Read the model definition and answer for the solid it produces. Units are mm, in the model's axes. A direction names the side the tool comes from. Give positions to 0.01 mm unless a question says otherwise; leave off trailing zeros. Order: outer loops, then holes, each group sorted by start corner. A loop starts at its lowest first (then second) coordinate and runs counter-clockwise, first axis right, second up.
Item 1: A cutting plane is placed at B-B (x = -72.5). Write down the section's boundary in (y, z).
Item 2: The mould has two halves that part along X. Classify faces 4 (the face through (-147.5, 6.18, -0.16)), 5 (the face through (-2, 0, 0)), 6 (the face through (141, 1.5, 0)): +X half, -X half, draft (parallel to the pull), parting line (faces both ways), or undercut.
Item 3: Given pin 1 Ø5 at (y, z) = (8, -3.5) entering from -X; pin 2 Ø1 at (x, y) = (-93.5, 2.5) entering from -Z; pin 3 Ø6 at (x, z) = (135.5, 1.5) entering from +Y, each flat-ended and moving along its own axis, determine where each tip first touches the part or whether it passes through.
Item 4: Which of the six approach directions +Z, -Z, +X, -X, +Y, -Y give full straight-line access (tool end or side, diameter ignored) to faces 1 (the face through (2, 6, -7.5)), 2 (the face through (147.5, 6.18, 0.16)), 3 (the face through (146.445, 6.923, -0.846))?
Item 5: A cutting plane is placed at A-A (y = 6.5). Write down the section's boundary in (x, z).
Item 6: Find the intervals of material crossed by line 1 along X through (y, z) = (9.75, 0); line 2 along Z through (x, y) = (-78.5, 6.5); line 3 along X through (y, z) = (1.25, 0), in increasing order.
from build123d import *

# Parameters (mm, degrees)
BOSS_EXTRUDE1_DEPTH = 1.5
SKETCH2_R           = 6.5
BOSS_EXTRUDE2_DEPTH = 10
BOSS_EXTRUDE3_DEPTH = 1
FILLET1_R           = 2
FILLET2_R           = 1
FILLET3_R           = 1
CUT_EXTRUDE1_DEPTH  = 151.73486657
SKETCH5_R           = 0.75
CUT_EXTRUDE2_DEPTH  = 151.73486657


with BuildPart() as part:
    # Sketch1 → Boss-Extrude1 (new body)
    with BuildSketch(Plane(origin=(0, 0, 0), x_dir=(1, 0, 0), z_dir=(0, 1, 0))):
        with BuildLine():
            Line((140, 7.5), (-140, 7.5))
            ThreePointArc((-140, 7.5), (-147.5, 0), (-140, -7.5))
            Line((-140, -7.5), (140, -7.5))
            ThreePointArc((140, -7.5), (147.5, 0), (140, 7.5))
        make_face()
    extrude(amount=BOSS_EXTRUDE1_DEPTH)

    # Sketch2 → Boss-Extrude2 (add)
    with BuildSketch(Plane(origin=(0, 1.5, 0), x_dir=(1, 0, 0), z_dir=(0, 1, 0))):
        with BuildLine():
            Line((-140, -7.5), (140, -7.5))
            ThreePointArc((140, -7.5), (147.5, 0), (140, 7.5))
            Line((140, 7.5), (-140, 7.5))
            ThreePointArc((-140, 7.5), (-147.5, 0), (-140, -7.5))
        make_face()
        with Locations(Location((140, 0, 0), (0, 0, 270))):
            Circle(SKETCH2_R, mode=Mode.SUBTRACT)
        with BuildLine():
            Line((-140, 6.5), (136.258342613, 6.5))
            ThreePointArc((136.258342613, 6.5), (132.5, 0), (136.258342613, -6.5))
            Line((136.258342613, -6.5), (-140, -6.5))
            ThreePointArc((-140, -6.5), (-146.5, 0), (-140, 6.5))
        make_face(mode=Mode.SUBTRACT)
    extrude(amount=BOSS_EXTRUDE2_DEPTH)

    # Sketch3 → Boss-Extrude3 (add)
    with BuildSketch(Plane(origin=(0, 11.5, 0), x_dir=(1, 0, 0), z_dir=(0, 1, 0))):
        with BuildLine():
            Line((-140, 10), (140, 10))
            ThreePointArc((140, 10), (150, 0), (140, -10))
            Line((140, -10), (-140, -10))
            ThreePointArc((-140, -10), (-150, 0), (-140, 10))
        make_face()
        with BuildLine():
            Line((-140, -6.5), (136.258342613, -6.5))
            Line((136.258342613, -6.5), (140, -6.5))
            ThreePointArc((140, -6.5), (146.5, 0), (140, 6.5))
            Line((140, 6.5), (136.258342613, 6.5))
            Line((136.258342613, 6.5), (-140, 6.5))
            ThreePointArc((-140, 6.5), (-146.5, 0), (-140, -6.5))
        make_face(mode=Mode.SUBTRACT)
    extrude(amount=BOSS_EXTRUDE3_DEPTH)

    # Fillet1
    # the kernel refuses this fillet: 2 mm, written as the material it takes off along each edge
    with BuildSketch(Plane(origin=(-140, 12.5, 0), x_dir=(0, 0, 1), z_dir=(1, 0, 0))) as fillet1_piece_1:
        with BuildLine():
            CenterArc((8.267949192, 2), FILLET1_R, 270, 60)
            Line((10, 1), (10.034641016, 0.98))
            ThreePointArc((10.034641016, 0.98), (10.04, 0.5), (10.04, 0))
            Line((10.04, 0), (10, -0.04))
            Line((10, -0.04), (8.267949192, -0.04))
            Line((8.267949192, -0.04), (8.267949192, 0))
        make_face()
    revolve(axis=Axis((-140, 12.5, 0), (0, -1, 0)), revolution_arc=180, mode=Mode.SUBTRACT)
    with BuildSketch(Plane(origin=(140, 12.5, 10), x_dir=(0, -1, 0), z_dir=(-1, 0, 0))) as fillet1_piece_2:
        with BuildLine():
            CenterArc((2, -1.732050808), FILLET1_R, 120, 60)
            Line((0, -1.732050808), (-0.04, -1.732050808))
            Line((-0.04, -1.732050808), (-0.04, 0))
            Line((-0.04, 0), (0, 0.04))
            ThreePointArc((0, 0.04), (0.5, 0.04), (0.98, 0.034641016))
            Line((0.98, 0.034641016), (1, 0))
        make_face()
    extrude(amount=280, mode=Mode.SUBTRACT)
    with BuildSketch(Plane(origin=(140, 12.5, 0), x_dir=(0, 0, -1), z_dir=(-1, 0, 0))) as fillet1_piece_3:
        with BuildLine():
            CenterArc((8.267949192, 2), FILLET1_R, 270, 60)
            Line((10, 1), (10.034641016, 0.98))
            ThreePointArc((10.034641016, 0.98), (10.04, 0.5), (10.04, 0))
            Line((10.04, 0), (10, -0.04))
            Line((10, -0.04), (8.267949192, -0.04))
            Line((8.267949192, -0.04), (8.267949192, 0))
        make_face()
    revolve(axis=Axis((140, 12.5, 0), (0, -1, 0)), revolution_arc=180, mode=Mode.SUBTRACT)
    with BuildSketch(Plane(origin=(-140, 12.5, -10), x_dir=(0, 0, 1), z_dir=(1, 0, 0))) as fillet1_piece_4:
        with BuildLine():
            CenterArc((1.732050808, 2), FILLET1_R, 210, 60)
            Line((0, 1), (-0.034641016, 0.98))
            ThreePointArc((-0.034641016, 0.98), (-0.04, 0.5), (-0.04, 0))
            Line((-0.04, 0), (0, -0.04))
            Line((0, -0.04), (1.732050808, -0.04))
            Line((1.732050808, -0.04), (1.732050808, 0))
        make_face()
    extrude(amount=280, mode=Mode.SUBTRACT)

    # Fillet2
    fillet2_edges = [part.edges().sort_by_distance(p)[0] for p in [
        (0, 0, -7.5),
        (147.5, 0, 0),
        (0, 0, 7.5),
        (-147.5, 0, 0),
    ]]
    fillet(fillet2_edges, radius=FILLET2_R)

    # Fillet3
    fillet3_edges = [part.edges().sort_by_distance(p)[0] for p in [
        (-146.5, 1.5, 0),
        (-1.870828693, 1.5, 6.5),
        (-1.870828693, 1.5, -6.5),
    ]]
    fillet(fillet3_edges, radius=FILLET3_R)

    # Sketch4 → Cut-Extrude1 (cut, through all)
    with BuildSketch(Plane(origin=(0, 1.5, 0), x_dir=(1, 0, 0), z_dir=(0, 1, 0))):
        with BuildLine():
            Line((-123.5, 3.5), (-103.5, 3.5))
            ThreePointArc((-103.5, 3.5), (-100, 0), (-103.5, -3.5))
            Line((-103.5, -3.5), (-123.5, -3.5))
            ThreePointArc((-123.5, -3.5), (-127, 0), (-123.5, 3.5))
        make_face()
    extrude(amount=-CUT_EXTRUDE1_DEPTH, mode=Mode.SUBTRACT)

    # Sketch5 → Cut-Extrude2 (cut, through all)
    with BuildSketch(Plane(origin=(0, 1.5, 0), x_dir=(1, 0, 0), z_dir=(0, 1, 0))):
        with Locations(Location((140, 0, 0), (0, 0, 270))):
            Circle(SKETCH5_R)
    extrude(amount=-CUT_EXTRUDE2_DEPTH, mode=Mode.SUBTRACT)


solid = part.part
Response values:
1. outline: (0, -6.5) arc R1 ccw to (1, -7.5) - (11.5, -7.5) - (11.5, -10) arc R2 ccw to (12.5, -8.27) - (12.5, -6.5) - (2.5, -6.5) arc R1 cw to (1.5, -5.5) - (1.5, 5.5) arc R1 cw to (2.5, 6.5) - (12.5, 6.5) - (12.5, 8.27) arc R2 ccw to (11.5, 10) - (11.5, 7.5) - (1, 7.5) arc R1 ccw to (0, 6.5) - close
2. face 4: -X half
2. face 5: draft
2. face 6: undercut
3. pin 1: stops at x = -147.43
3. pin 2: stops at z = -7.5
3. pin 3: stops at y = 11.5
4. face 1: -Z, +X, -X, -Y
4. face 2: +X, -Y
4. face 3: +Y
5. outline: (-140, -7.5) - (140, -7.5) arc R7.5 ccw to (140, 7.5) - (-140, 7.5) arc R7.5 ccw to start; hole (-140, -6.5) - (136.26, -6.5) arc R7.5 cw to (136.26, 6.5) - (-140, 6.5) arc R6.5 ccw to start; hole circle Ø13 at (140, 0)
6. line 1: x = -147.5 to -146.5, 132.5 to 133.5, 146.5 to 147.5
6. line 2: z = -7.5 to -6.5, 6.5 to 7.5
6. line 3: x = -147.5 to -127, -100 to 139.25, 140.75 to 147.5
